from build123d import *

# Parameters (mm, degrees)
F0_W     = 76.2
F0_H     = 76.2
F0_W_2   = 50.8
F0_H_2   = 50.8
F1_DEPTH = 6.35
F2_DEPTH = 19.05
F3_R     = 1.5875
F4_DEPTH = 25.4
F5_R     = 3.175
F6_DEPTH = 19.051


with BuildPart() as f1:
    # F0 (on Top) → F1 (new body)
    with BuildSketch(Plane.XY):
        Rectangle(F0_W, F0_H)
        Rectangle(F0_W_2, F0_H_2, mode=Mode.SUBTRACT)
        Rectangle(F0_W_2, F0_H_2)
    extrude(amount=F1_DEPTH)

    # F0 (on Top) → F2 (join)
    with BuildSketch(Plane.XY):
        Rectangle(F0_W, F0_H)
        Rectangle(F0_W_2, F0_H_2, mode=Mode.SUBTRACT)
    extrude(amount=F2_DEPTH)

    # F3 (on face) → F4 (cut)
    with BuildSketch(Plane(origin=(0, 38.1, 0), x_dir=(-1, 0, 0), z_dir=(0, 1, 0))):
        with Locations((0, 13.97)):
            Circle(F3_R)
    extrude(amount=-F4_DEPTH, mode=Mode.SUBTRACT)

    # F5 (on face) → F6 (cut, through all)
    with BuildSketch(Plane.XY.offset(19.05)):
        with Locations((-31.75, 31.75)):
            Circle(F5_R)
        with Locations((31.75, 31.75)):
            Circle(F5_R)
        with Locations((31.75, -31.75)):
            Circle(F5_R)
        with Locations((-31.75, -31.75)):
            Circle(F5_R)
    extrude(amount=-F6_DEPTH, mode=Mode.SUBTRACT)


solid = f1.part
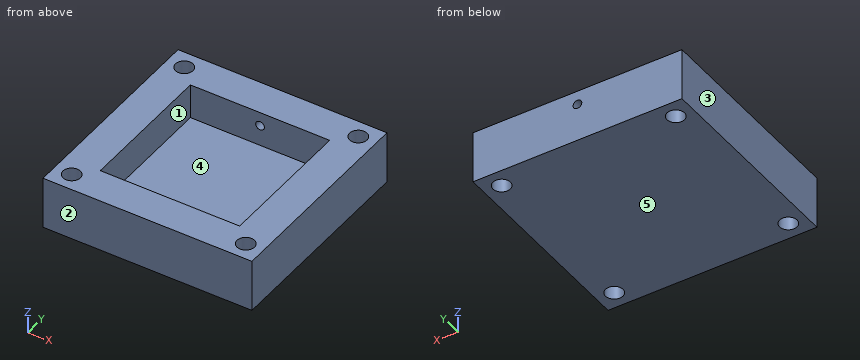
Model file for the job. Use its own axes, mm. Face numbers are marked on the shaded views. A direction names the side the tool comes from. Give positions to 0.01 mm unless a question says otherwise; leave off trailing zeros. Loops run counter-clockwise (first coordinate to the right, second up) from the corner with the lowest first, then second, coordinate; pieces in that order, holes last.
Item 1: Slice it at C-C (x = 0). Write the cut outline in (y, z), plus the area to 3 significant figures.
Check values:
outline: (-38.1, 0) - (38.1, 0) - (38.1, 12.38) - (25.4, 12.38) - (25.4, 6.35) - (-25.4, 6.35) - (-25.4, 19.05) - (-38.1, 19.05) - close; (25.4, 15.56) - (38.1, 15.56) - (38.1, 19.05) - (25.4, 19.05) - close
area: 766 mm2
Item 2: Slice it at B-B (y = 31.75). Give the number of separate pieces and of enclosed holes in the cut face, plus the area to 3 significant figures.
Check values:
separate pieces: 3
enclosed holes: 1
area: 1,200 mm2
Item 3: Drop a flat-ended pin along its axis: P1, Ø8, axis at x = -8, y = -9.5, coming from the +Z side. Give the stop position or say it passes through.
Check values:
P1: stops at z = 6.35
Item 4: Mould opens along X. For the marked faces 1, 2 and 3 say: +X half, -X half, draft (parallel to the pull), parting line (faces both ways), or undercut.
Check values:
face 1: undercut
face 2: draft
face 3: -X half
Item 5: Slice it at D-D (z = 17). Write the cut outline in (x, y) (3 decimals), plus the area to 3 significant figures.
Check values:
outline: (-38.1, -38.1) - (38.1, -38.1) - (38.1, 38.1) - (-38.1, 38.1) - close; hole circle Ø6.35 at (-31.75, -31.75); hole circle Ø6.35 at (-31.75, 31.75); hole (-25.4, -25.4) - (25.4, -25.4) - (25.4, 25.4) - (-25.4, 25.4) - close; hole circle Ø6.35 at (31.75, -31.75); hole circle Ø6.35 at (31.75, 31.75)
area: 3,100 mm2
Item 6: Slice it at A-A (z = 2.5). Write the cut outline in (x, y) (3 decimals).
Check values:
outline: (-38.1, -38.1) - (38.1, -38.1) - (38.1, 38.1) - (-38.1, 38.1) - close; hole circle Ø6.35 at (-31.75, -31.75); hole circle Ø6.35 at (-31.75, 31.75); hole circle Ø6.35 at (31.75, -31.75); hole circle Ø6.35 at (31.75, 31.75)
Item 7: Which spindle directions (+Z, -Z, +X, -X, +Y, -Y) get a long thin tool onto all of the face, cutting with end or side? Do the marked faces 4 and 5. Say none if no direction does.
Check values:
face 4: +Z
face 5: -Z, +X, -X, +Y, -Y
Item 8: Drill centre lines: line 1 along Y through (x, z) = (-31.75, 6) (3 decimals); line 2 along X through (y, z) = (24, 17). Where is each one in solid material? Low to high.
Check values:
line 1: y = -38.1 to -34.925, -28.575 to 28.575, 34.925 to 38.1
line 2: x = -38.1 to -25.4, 25.4 to 38.1
